Geometry: final body of the model. Coordinates: model frame, mm. A direction names the side the tool comes from. Give positions to 0.01 mm unless a question says otherwise; leave off trailing zeros. Order: outer loops, then holes, each group sorted by start corner. A loop starts at its lowest first (then second) coordinate and runs counter-clockwise, first axis right, second up. Notation, with made-up numbers: (60, -9.5) -> (84, -9.5) arc R14 ccw to (84, 9.5) -> close; hole circle Ø10 at (-36, -13.75). An arc over 180 degrees is marked (long way). Write item = value, one per line.
```python
from build123d import *

# Parameters (mm, degrees)
BOSS_EXTRUDE1_DEPTH              = 25.4
F_1_2_13_TAPPED_HOLE1_AT_2_COUNT = 2
F_1_2_13_TAPPED_HOLE1_AT_2_PITCH = 95.25
CUT_EXTRUDE1_DEPTH               = 5.842
CUT_EXTRUDE2_DEPTH               = 1.016
F_3_8_16_TAPPED_HOLE1_AT_2_COUNT = 2
F_3_8_16_TAPPED_HOLE1_AT_2_PITCH = 27.94
CUT_EXTRUDE3_DEPTH               = 26.4
CUT_EXTRUDE4_DEPTH               = 10.668
SKETCH15_W                       = 19.05
SKETCH15_H                       = 16.51
CUT_EXTRUDE5_DEPTH               = 119.11


with BuildPart() as part:
    # Sketch6 → Boss-Extrude1 (new body)
    with BuildSketch(Plane.XY):
        Polygon((-36.576, 59.055), (57.15, 59.055), (58.674, 57.531), (58.674, -57.531), (57.15, -59.055), (-36.576, -59.055), (-38.1, -57.531), (-38.1, 57.531), align=None)
    extrude(amount=-BOSS_EXTRUDE1_DEPTH)

    # Sketch7 → 1/2-13 Tapped Hole1 (revolve, cut)
    with BuildSketch(Plane(origin=(0, 47.625, -25.4), x_dir=(0, 1, 0), z_dir=(1, 0, 0))):
        Polygon((0, 0), (0, 25.4), (6.985, 25.4), (6.35, 24.765), (6.35, 0.635), (6.985, 0), align=None)
    f_1_2_13_tapped_hole1 = revolve(axis=Axis((0, 47.625, -31.75), (0, 0, 1)), mode=Mode.SUBTRACT)

    # 1/2-13 Tapped Hole1 at 2: 1/2-13 Tapped Hole1 ×2
    with Locations(*[(0, -i * F_1_2_13_TAPPED_HOLE1_AT_2_PITCH, 0) for i in range(1, F_1_2_13_TAPPED_HOLE1_AT_2_COUNT)]):
        add(f_1_2_13_tapped_hole1, mode=Mode.SUBTRACT)

    # Sketch9 → Cut-Extrude1 (cut)
    with BuildSketch(Plane(origin=(0, 0, 0), x_dir=(-1, 0, 0), z_dir=(0, 0, -1))):
        with BuildLine():
            Line((-2.413, 17.78), (-2.413, 36.83))
            ThreePointArc((-2.413, 36.83), (0, 39.243), (2.413, 36.83))
            Line((2.413, 36.83), (2.413, 17.78))
            ThreePointArc((2.413, 17.78), (0, 15.367), (-2.413, 17.78))
        make_face()
        with BuildLine():
            Line((2.413, -17.78), (2.413, -36.83))
            ThreePointArc((2.413, -36.83), (0, -39.243), (-2.413, -36.83))
            Line((-2.413, -36.83), (-2.413, -17.78))
            ThreePointArc((-2.413, -17.78), (0, -15.367), (2.413, -17.78))
        make_face()
    extrude(amount=CUT_EXTRUDE1_DEPTH, mode=Mode.SUBTRACT)

    # Sketch12 → Cut-Extrude2 (cut)
    with BuildSketch(Plane.XY):
        Polygon((38.1, 57.531), (38.1, -57.531), (36.576, -59.055), (57.15, -59.055), (58.674, -57.531), (58.674, 57.531), (57.15, 59.055), (36.576, 59.055), align=None)
    extrude(amount=-CUT_EXTRUDE2_DEPTH, mode=Mode.SUBTRACT)

    # Sketch10 → 3/8-16 Tapped Hole1 (revolve, cut)
    with BuildSketch(Plane(origin=(58.674, 13.97, -13.208), x_dir=(0, 0, -1), z_dir=(0, 1, 0))):
        Polygon((0, 0), (0, 27.987865582), (3.96875, 25.6032), (3.96875, 21.59), (4.7625, 21.59), (4.7625, 0.635), (5.3975, 0), align=None)
    f_3_8_16_tapped_hole1 = revolve(axis=Axis((65.024, 13.97, -13.208), (-1, 0, 0)), mode=Mode.SUBTRACT)

    # 3/8-16 Tapped Hole1 at 2: 3/8-16 Tapped Hole1 ×2
    with Locations(*[(0, -i * F_3_8_16_TAPPED_HOLE1_AT_2_PITCH, 0) for i in range(1, F_3_8_16_TAPPED_HOLE1_AT_2_COUNT)]):
        add(f_3_8_16_tapped_hole1, mode=Mode.SUBTRACT)

    # Sketch13 → Cut-Extrude3 (cut, through all)
    with BuildSketch(Plane.XY):
        with BuildLine():
            Line((28.7782, 47.625), (28.7782, 28.575))
            ThreePointArc((28.7782, 28.575), (25.4, 25.1968), (22.0218, 28.575))
            Line((22.0218, 28.575), (22.0218, 47.625))
            ThreePointArc((22.0218, 47.625), (25.4, 51.0032), (28.7782, 47.625))
        make_face()
        with BuildLine():
            Line((28.7782, -28.575), (28.7782, -47.625))
            ThreePointArc((28.7782, -47.625), (25.4, -51.0032), (22.0218, -47.625))
            Line((22.0218, -47.625), (22.0218, -28.575))
            ThreePointArc((22.0218, -28.575), (25.4, -25.1968), (28.7782, -28.575))
        make_face()
    extrude(amount=-CUT_EXTRUDE3_DEPTH, mode=Mode.SUBTRACT)

    # Sketch14 → Cut-Extrude4 (cut)
    with BuildSketch(Plane.XY.offset(-25.4)):
        with BuildLine():
            Line((32.54375, 47.625), (32.54375, 28.575))
            ThreePointArc((32.54375, 28.575), (25.4, 21.43125), (18.25625, 28.575))
            Line((18.25625, 28.575), (18.25625, 47.625))
            ThreePointArc((18.25625, 47.625), (25.4, 54.76875), (32.54375, 47.625))
        make_face()
        with BuildLine():
            Line((32.54375, -28.575), (32.54375, -47.625))
            ThreePointArc((32.54375, -47.625), (25.4, -54.76875), (18.25625, -47.625))
            Line((18.25625, -47.625), (18.25625, -28.575))
            ThreePointArc((18.25625, -28.575), (25.4, -21.43125), (32.54375, -28.575))
        make_face()
    extrude(amount=CUT_EXTRUDE4_DEPTH, mode=Mode.SUBTRACT)

    # Sketch15 → Cut-Extrude5 (cut, through all)
    with BuildSketch(Plane.XZ.offset(59.055)):
        with Locations((-28.575, -17.145)):
            Rectangle(SKETCH15_W, SKETCH15_H)
    extrude(amount=-CUT_EXTRUDE5_DEPTH, mode=Mode.SUBTRACT)


solid = part.part
```
1) Section query A-A (z = -3.75). Output: boundary loops of the cut face in (x, y) (3 decimals).
Check sheet entries:
outline = (-38.1, -57.531) -> (-36.576, -59.055) -> (57.15, -59.055) -> (58.674, -57.531) -> (58.674, 57.531) -> (57.15, 59.055) -> (-36.576, 59.055) -> (-38.1, 57.531) -> close; hole circle Ø12.7 at (0, -47.625); hole circle Ø12.7 at (0, 47.625); hole (-2.413, -36.83) arc R2.413 ccw to (2.413, -36.83) -> (2.413, -17.78) arc R2.413 ccw to (-2.413, -17.78) -> close; hole (-2.413, 17.78) arc R2.413 ccw to (2.413, 17.78) -> (2.413, 36.83) arc R2.413 ccw to (-2.413, 36.83) -> close; hole (22.022, -47.625) arc R3.378 ccw to (28.778, -47.625) -> (28.778, -28.575) arc R3.378 ccw to (22.022, -28.575) -> close; hole (22.022, 28.575) arc R3.378 ccw to (28.778, 28.575) -> (28.778, 47.625) arc R3.378 ccw to (22.022, 47.625) -> close
2) First-contact query: P1, Ø9.5, axis at x = -28.5, y = -4, coming from the -Z side; P2, Ø8.5, axis at y = 34.5, z = -18.5, coming from the -X side; P3, Ø4.5, axis at x = 28, y = 30, coming from the -Z side. Flat tips, straight axial feed; report the tip coordinate or a pass-through.
Check sheet entries:
P1 = -8.89
P2 = -19.05
P3 = -14.73
3) Mould query, pull axis X, two halves, no side actions, for faces 1 (the face through (20, 1, -25.4)), 2 (the face through (-0.053, -39.242, -2.88)), 3 (the face through (-38.1, -1, -4)). Classes: +X half, -X half, draft (parallel to the pull), parting line (faces both ways), or undercut.
Check sheet entries:
face_1 = draft
face_2 = undercut
face_3 = -X half
4) Section query D-D (z = -20). Count the separate pieces of the cut face and the enclosed holes in it, plus the area to 3 significant figures.
Check sheet entries:
separate_pieces = 1
enclosed_holes = 4
area = 8,060 mm²
5) Reachability of faces 4 (the face through (0, 27, -5.842)), 5 (the face through (22.022, 38, -7)), 6 (the face through (1, 1, 0)), 7 (the face through (47.71, 15.79, -17.61)), 8 (the face through (30, 38, -14.732)) from +Z, -Z, +X, -X, +Y, -Y: full face, straight path, thin tool, end or side. Return the list, or none.
Check sheet entries:
face_4 = +Z
face_5 = +Z, -Z
face_6 = +Z, +X, -X, +Y, -Y
face_7 = +X
face_8 = -Z
6) Section query B-B (x = 25.4). Output: boundary loops of the cut face in (y, z) (3 decimals).
Check sheet entries:
outline = (-59.055, -25.4) -> (-54.769, -25.4) -> (-54.769, -14.732) -> (-51.003, -14.732) -> (-51.003, 0) -> (-59.055, 0) -> close; (-25.197, -14.732) -> (-21.431, -14.732) -> (-21.431, -25.4) -> (21.431, -25.4) -> (21.431, -14.732) -> (25.197, -14.732) -> (25.197, 0) -> (-25.197, 0) -> close; (51.003, -14.732) -> (54.769, -14.732) -> (54.769, -25.4) -> (59.055, -25.4) -> (59.055, 0) -> (51.003, 0) -> close
7) Section query C-C (y = -27). Output: boundary loops of the cut face in (x, z), plus the area to 3 significant figures.
Check sheet entries:
outline = (-38.1, -8.89) -> (-19.05, -8.89) -> (-19.05, -25.4) -> (18.43, -25.4) -> (18.43, -14.73) -> (22.41, -14.73) -> (22.41, 0) -> (2.41, 0) -> (2.41, -5.84) -> (-2.41, -5.84) -> (-2.41, 0) -> (-38.1, 0) -> close; (28.39, -14.73) -> (32.37, -14.73) -> (32.37, -25.4) -> (58.67, -25.4) -> (58.67, -1.02) -> (38.1, -1.02) -> (38.1, 0) -> (28.39, 0) -> close
area = 1,860 mm²
8) Line query: line 1 (Y direction, x = 0, z = -19.5) (3 decimals); line 2 (Z direction, x = 36.3, y = 13.97); line 3 (Y direction, x = 1.5, z = -12.5) (3 decimals). Output: solid intervals per line, ascending. Write a range as from..to.
Check sheet entries:
line_1 = -59.055..-53.975, -41.275..41.275, 53.975..59.055
line_2 = -25.4..-17.18, -9.24..0
line_3 = -59.055..-53.795, -41.455..41.455, 53.795..59.055
